```python
from build123d import *

# Parameters (mm, degrees)
F1_R     = 7.4238247782
F3_W     = 24.2328178138
F3_H     = 90.0287199765
F3_W_2   = 11.5328170359
F3_H_2   = 77.3287191987
F4_DEPTH = 63.5
F4_TAPER = -3


with BuildPart() as f2:
    # F2: sweep along a path in F0
    with BuildLine(Plane.XZ) as f2_path:
        Line((0, 0), (18.8963264227, 0))
        Line((18.8963264227, 0), (30.0118159503, 25.0590108335))
        Line((30.0118159503, 25.0590108335), (36.1253321171, 12.3736970127))
        Line((36.1253321171, 12.3736970127), (46.6850474477, 23.2028663158))
        Line((46.6850474477, 23.2028663158), (46.6850474477, 0))
        Line((46.6850474477, 0), (68.916015327, 0))
    # F1 (on Right) → F2 (sweep)
    with BuildSketch(Plane.YZ):
        Circle(F1_R)
    sweep(path=f2_path.line, transition=Transition.RIGHT)

    # F3 (on Right) → F4 (cut, symmetric)
    with BuildSketch(Plane.YZ):
        Rectangle(F3_W, F3_H)
        Rectangle(F3_W_2, F3_H_2, mode=Mode.SUBTRACT)
    extrude(amount=F4_DEPTH, both=True, taper=F4_TAPER, mode=Mode.SUBTRACT)


solid = f2.part
```
Design review of the part built by this model. Coordinates are the model's own, in mm. A direction names the side the tool comes from. Round coordinates to 2 decimals unless told otherwise and drop trailing zeros.
Item 1: Clearance check with flat-ended pins moving along their axes: pin 1 Ø4 at (x, y) = (44, 2.5) entering from +Z; pin 2 Ø12 at (x, z) = (50, 32.5) entering from +Y; pin 3 Ø12 at (x, z) = (40.5, 31.5) entering from -Y. State where each tip first meets the part, or that it passes through.
Item 2: For probe 1 along X at (y, z) = (-1.25, 1); probe 2 along Z at (x, y) = (12, -0.5); probe 3 along X at (y, z) = (-1.75, 26.5), list the stretches that pass through material, from the lowest coordinate up.
Item 3: The part is to be moulded in two halves that separate along X. For faces 1 (the flat face through (68.916, 0, 0)), 2 (the cylindrical face through (20.63, 0.08, 22.22)), 3 (the cylindrical face through (35.58, 0.06, 30.6)), say which applies: +X half, -X half, draft (parallel to the pull), parting line (faces both ways), or undercut.
Item 4: For faces 4 (the cylindrical face through (54.11, 0.04, 21.13)), 5 (the cylindrical face through (6.06, 0.092, 7.423)), 6 (the cylindrical face through (60.886, -1.609, -7.247)), 7 (the cylindrical face through (37.53, -0.06, 3.18)), list the 3-axis set-ups (+Z, -Z, +X, -X, +Y, -Y) from which the entire face can be reached by the end or side of a thin tool; tool diameter is ignored.
Returned:
1. pin 1: stops at z = 32.69
1. pin 2: stops at y = 3.44
1. pin 3: stops at y = -3.94
2. probe 1: x = 0 to 27.35, 33.48 to 35.26, 39.37 to 68.92
2. probe 2: z = -7.41 to 7.41
2. probe 3: x = 22.76 to 37.33, 39.82 to 53.9
3. face 1: +X half
3. face 2: -X half
3. face 3: undercut
4. face 4: +Z, +X
4. face 5: +Z, -X
4. face 6: +X
4. face 7: -Z
